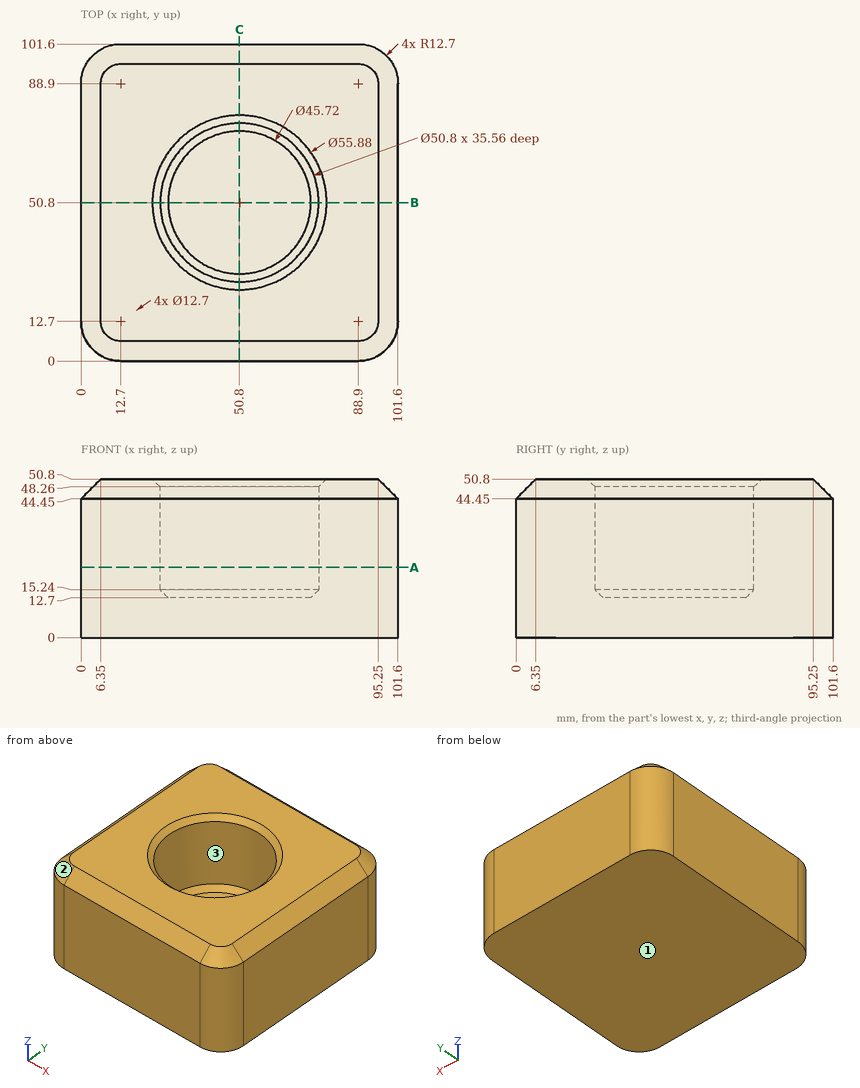
For this review, use the dimensioned drawing (mm, ordinates from the lowest corner) and the shaded views. Give positions to 0.01 mm unless a question says otherwise; leave off trailing zeros. Loops run counter-clockwise (first coordinate to the right, second up) from the corner with the lowest first, then second, coordinate; pieces in that order, holes last.
Item 1: Take a section at B-B, the plane y = 50.8. State the section outline as (x, z) points, and give its area (3 significant figures).
Item 2: Draft analysis for pull direction Y (two halves, no side actions). For the marked faces 1, 2 and 3, state which applies: +Y half, -Y half, draft (parallel to the pull), parting line (faces both ways), or undercut.
Item 3: For line 1 along Y through (x, z) = (50.8, 27.5); line 2 along X through (y, z) = (50, 32); line 3 along X through (y, z) = (70, 34.5), list the stretches that pass through material, from the lowest coordinate up.
Item 4: Insertion check: pin 1 (13.5 mm diameter, centred on x = 60, y = 47, fed in from +Z); pin 2 (5 mm diameter, centred on x = 82, z = 26.5, fed in from -Y). Each pin has a flat end and moves straight along its axis. Give the tip position at first contact, or say it passes through.
Item 5: Take a section at A-A, the plane z = 22.5. State the section outline as (x, y) points, and give its area (3 significant figures).
Calculated:
1. outline: (0, 0) - (101.6, 0) - (101.6, 44.45) - (95.25, 50.8) - (78.74, 50.8) - (76.2, 48.26) - (76.2, 15.24) - (73.66, 12.7) - (27.94, 12.7) - (25.4, 15.24) - (25.4, 48.26) - (22.86, 50.8) - (6.35, 50.8) - (0, 44.45) - close
1. area: 3,190 mm2
2. face 1: draft
2. face 2: -Y half
2. face 3: undercut
3. line 1: y = 0 to 25.4, 76.2 to 101.6
3. line 2: x = 0 to 25.41, 76.19 to 101.6
3. line 3: x = 0 to 34.17, 67.43 to 101.6
4. pin 1: stops at z = 12.7
4. pin 2: stops at y = 0
5. outline: (0, 12.7) arc R12.7 ccw to (12.7, 0) - (88.9, 0) arc R12.7 ccw to (101.6, 12.7) - (101.6, 88.9) arc R12.7 ccw to (88.9, 101.6) - (12.7, 101.6) arc R12.7 ccw to (0, 88.9) - close; hole circle Ø50.8 at (50.8, 50.8)
5. area: 8,160 mm2
